Can you work these out from the model? Positions are in its coordinate system, mm. Face numbers are marked on the shaded views. A direction names the side the tool comes from. Coordinates: 2 decimals unless noted, no trailing zeros. Loops run counter-clockwise (first coordinate to the right, second up) from the corner with the lowest first, then second, coordinate; pieces in that order, holes last.
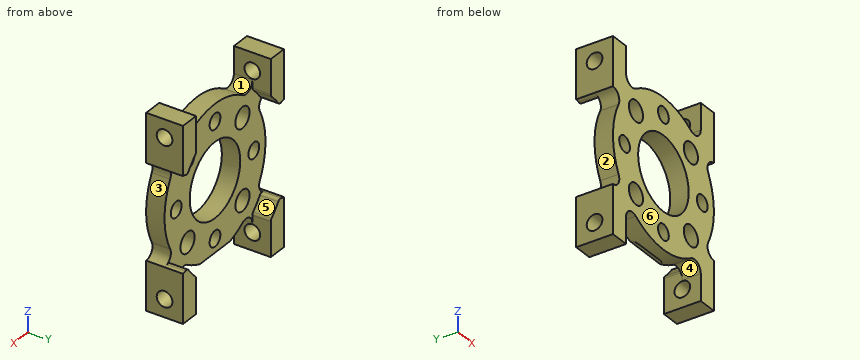
```python
from build123d import *

# Parameters (mm, degrees)
CUT_EXTRUDE1_START         = -6.35
CUT_EXTRUDE1_DEPTH         = 3.175
CUT_EXTRUDE1_START_2       = -3.175
CUT_EXTRUDE1_2_DEPTH       = 3.175
SKETCH2_W                  = 3.293618
SKETCH2_H                  = 6.35
BOSS_EXTRUDE1_DEPTH        = 4.551833731
SKETCH3_W                  = 3.293618
SKETCH3_H                  = 6.35
BOSS_EXTRUDE2_DEPTH        = 4.551833731
SKETCH4_W                  = 3.293618
SKETCH4_H                  = 6.35
BOSS_EXTRUDE3_DEPTH        = 4.551833731
SKETCH5_W                  = 3.293618
SKETCH5_H                  = 6.35
BOSS_EXTRUDE4_DEPTH        = 4.551833731
HOLE1_D                    = 12.7254
M2_5_CLEARANCE_HOLE1_D     = 2.7051
M3_CLEARANCE_HOLE1_D       = 3.556
M2_5_CLEARANCE_HOLE2_D     = 2.7051
M2_5_CLEARANCE_HOLE2_DEPTH = 3.293618
M2_5_CLEARANCE_HOLE3_D     = 2.7051
M2_5_CLEARANCE_HOLE3_DEPTH = 3.293618
M2_5_CLEARANCE_HOLE4_D     = 2.7051
M2_5_CLEARANCE_HOLE4_DEPTH = 25.4
M2_5_CLEARANCE_HOLE5_D     = 2.7051
M2_5_CLEARANCE_HOLE5_DEPTH = 3.293618
FILLET1_R                  = 0.635


with BuildPart() as part:
    # Cut-Extrude1: read off the stored shape, not the designer's step
    # Cut-Extrude1 outline → Cut-Extrude1 (new body)
    with BuildSketch(Plane(origin=(0, 6.35, 0), x_dir=(-1, 0, 0), z_dir=(0, 1, 0)).offset(CUT_EXTRUDE1_START)):
        with BuildLine():
            ThreePointArc((-12.7, 8.135112), (-11.343887812, 7.373541875), (-11.288347253, 5.819210969))
            ThreePointArc((-11.288347253, 5.819210969), (-12.7, 0), (-11.288347253, -5.819210969))
            ThreePointArc((-11.288347253, -5.819210969), (-11.343887812, -7.373541875), (-12.7, -8.135112))
            Line((-12.7, -8.135112), (-12.7, -11.958166269))
            Line((-12.7, -11.958166269), (-9.406382, -11.958166269))
            ThreePointArc((-9.406382, -11.958166269), (-8.574193969, -10.561863981), (-6.950117333, -10.629481128))
            ThreePointArc((-6.950117333, -10.629481128), (0, -12.7), (6.950117333, -10.629481128))
            ThreePointArc((6.950117333, -10.629481128), (8.574193969, -10.561863981), (9.406382, -11.958166269))
            Line((9.406382, -11.958166269), (12.7, -11.958166269))
            Line((12.7, -11.958166269), (12.7, -8.135112))
            ThreePointArc((12.7, -8.135112), (11.343887812, -7.373541875), (11.288347253, -5.819210969))
            ThreePointArc((11.288347253, -5.819210969), (12.7, 0), (11.288347253, 5.819210969))
            ThreePointArc((11.288347253, 5.819210969), (11.343887812, 7.373541875), (12.7, 8.135112))
            Line((12.7, 8.135112), (12.7, 11.958166269))
            Line((12.7, 11.958166269), (9.406382, 11.958166269))
            ThreePointArc((9.406382, 11.958166269), (8.574193969, 10.561863981), (6.950117333, 10.629481128))
            ThreePointArc((6.950117333, 10.629481128), (0, 12.7), (-6.950117333, 10.629481128))
            ThreePointArc((-6.950117333, 10.629481128), (-8.574193969, 10.561863981), (-9.406382, 11.958166269))
            Line((-9.406382, 11.958166269), (-12.7, 11.958166269))
            Line((-12.7, 11.958166269), (-12.7, 8.135112))
        make_face()
    extrude(amount=CUT_EXTRUDE1_DEPTH)

    # Cut-Extrude1 2 outline → Cut-Extrude1 2 (add)
    with BuildSketch(Plane(origin=(0, 6.35, 0), x_dir=(-1, 0, 0), z_dir=(0, 1, 0)).offset(CUT_EXTRUDE1_START_2)):
        with BuildLine():
            Line((-9.406382, 10.328643554), (-9.406382, 11.958166269))
            Line((-9.406382, 11.958166269), (-12.7, 11.958166269))
            Line((-12.7, 11.958166269), (-12.7, 8.135112))
            ThreePointArc((-12.7, 8.135112), (-12.131266538, 8.02978706), (-11.637967358, 7.727782073))
            ThreePointArc((-11.637967358, 7.727782073), (-10.602229958, 9.096901665), (-9.406382, 10.328643554))
        make_face()
        with BuildLine():
            Line((12.7, 11.958166269), (9.406382, 11.958166269))
            Line((9.406382, 11.958166269), (9.406382, 10.328643554))
            ThreePointArc((9.406382, 10.328643554), (10.602229958, 9.096901665), (11.637967358, 7.727782073))
            ThreePointArc((11.637967358, 7.727782073), (12.131266538, 8.02978706), (12.7, 8.135112))
            Line((12.7, 8.135112), (12.7, 11.958166269))
        make_face()
        with BuildLine():
            ThreePointArc((-9.406382, -10.328643554), (-10.602229958, -9.096901665), (-11.637967358, -7.727782073))
            ThreePointArc((-11.637967358, -7.727782073), (-12.131266538, -8.02978706), (-12.7, -8.135112))
            Line((-12.7, -8.135112), (-12.7, -11.958166269))
            Line((-12.7, -11.958166269), (-9.406382, -11.958166269))
            Line((-9.406382, -11.958166269), (-9.406382, -10.328643554))
        make_face()
        with BuildLine():
            ThreePointArc((12.7, -8.135112), (12.131266538, -8.02978706), (11.637967358, -7.727782073))
            ThreePointArc((11.637967358, -7.727782073), (10.602229958, -9.096901665), (9.406382, -10.328643554))
            Line((9.406382, -10.328643554), (9.406382, -11.958166269))
            Line((9.406382, -11.958166269), (12.7, -11.958166269))
            Line((12.7, -11.958166269), (12.7, -8.135112))
        make_face()
    extrude(amount=CUT_EXTRUDE1_2_DEPTH)

    # Sketch2 → Boss-Extrude1 (add)
    with BuildSketch(Plane(origin=(0, 0, -11.958166269), x_dir=(-1, 0, 0), z_dir=(0, 0, -1))):
        with Locations((11.053191, 3.175)):
            Rectangle(SKETCH2_W, SKETCH2_H)
    extrude(amount=BOSS_EXTRUDE1_DEPTH)

    # Sketch3 → Boss-Extrude2 (add)
    with BuildSketch(Plane(origin=(0, 0, -11.958166269), x_dir=(-1, 0, 0), z_dir=(0, 0, -1))):
        with Locations((-11.053191, 3.175)):
            Rectangle(SKETCH3_W, SKETCH3_H)
    extrude(amount=BOSS_EXTRUDE2_DEPTH)

    # Sketch4 → Boss-Extrude3 (add)
    with BuildSketch(Plane.XY.offset(11.958166269)):
        with Locations((11.053191, 3.175)):
            Rectangle(SKETCH4_W, SKETCH4_H)
    extrude(amount=BOSS_EXTRUDE3_DEPTH)

    # Sketch5 → Boss-Extrude4 (add)
    with BuildSketch(Plane.XY.offset(11.958166269)):
        with Locations((-11.053191, 3.175)):
            Rectangle(SKETCH5_W, SKETCH5_H)
    extrude(amount=BOSS_EXTRUDE4_DEPTH)

    # Hole1 (through all)
    with Locations(Plane(origin=(0, 3.175, 0), x_dir=(1, 0, 0), z_dir=(0, 1, 0))):
        with Locations((0, 0)):
            Hole(HOLE1_D / 2)

    # M2.5 Clearance Hole1 (through all)
    with Locations(Plane(origin=(0, 3.175, 0), x_dir=(1, 0, 0), z_dir=(0, 1, 0))):
        with Locations((0, -9.779), (-9.779, 0), (0, 9.779), (9.779, 0)):
            Hole(M2_5_CLEARANCE_HOLE1_D / 2)

    # M3 Clearance Hole1 (through all)
    with Locations(Plane(origin=(0, 3.175, 0), x_dir=(1, 0, 0), z_dir=(0, 1, 0))):
        with Locations((-6.914797213, -6.914797213), (-6.914797213, 6.914797213), (6.914797213, 6.914797213), (6.914797213, -6.914797213)):
            Hole(M3_CLEARANCE_HOLE1_D / 2)

    # M2.5 Clearance Hole2
    with Locations(Plane.ZY.offset(12.7)):
        with Locations((13.470384182, 3.175)):
            Hole(M2_5_CLEARANCE_HOLE2_D / 2, depth=M2_5_CLEARANCE_HOLE2_DEPTH)

    # M2.5 Clearance Hole3
    with Locations(Plane(origin=(-9.406382, 0, 0), x_dir=(0, 0, -1), z_dir=(1, 0, 0))):
        with Locations((13.470384182, 3.175)):
            Hole(M2_5_CLEARANCE_HOLE3_D / 2, depth=M2_5_CLEARANCE_HOLE3_DEPTH)

    # M2.5 Clearance Hole4
    with Locations(Plane(origin=(12.7, 0, 0), x_dir=(0, 0, -1), z_dir=(1, 0, 0))):
        with Locations((13.470384182, 3.175)):
            Hole(M2_5_CLEARANCE_HOLE4_D / 2, depth=M2_5_CLEARANCE_HOLE4_DEPTH)

    # M2.5 Clearance Hole5
    with Locations(Plane.ZY.offset(-9.406382)):
        with Locations((13.470384182, 3.175)):
            Hole(M2_5_CLEARANCE_HOLE5_D / 2, depth=M2_5_CLEARANCE_HOLE5_DEPTH)

    # Fillet1
    # the kernel refuses this fillet: 0.635 mm, written as the material it takes off along each edge
    with BuildSketch(Plane(origin=(-9.406382, 3.175, 10.328643554), x_dir=(0, 0, 1), z_dir=(0, 1, 0)), Plane(origin=(9.406382, 3.175, -10.328643554), x_dir=(0, 0, -1), z_dir=(0, 1, 0))) as fillet1_piece_1:
        with BuildLine():
            CenterArc((0.276858439, -0.635), FILLET1_R, 90, 46.565062077)
            ThreePointArc((-0.184250343, -0.198418174), (-0.091644431, -0.0996555), (0, 0))
            Line((0, 0), (0.276858439, 0))
        make_face()
    extrude(amount=3.867146097, mode=Mode.SUBTRACT)
    with BuildSketch(Plane(origin=(-11.637967358, 3.175, -7.727782073), x_dir=(0.5706588735868443, 0, -0.8211872198205438), z_dir=(0, 1, 0)), Plane(origin=(11.637967358, 3.175, 7.727782073), x_dir=(-0.5706588735868443, 0, 0.8211872198205438), z_dir=(0, 1, 0))) as fillet1_piece_2:
        with BuildLine():
            CenterArc((0.604132084, 0.634858067), FILLET1_R, 191.325534433, 77.463029076)
            ThreePointArc((-0.018502711, 0.51015477), (0.011380109, 0.255825664), (0, 0))
            ThreePointArc((0, 0), (0.295353463, 0.003122527), (0.590706926, 0))
        make_face()
    extrude(amount=4.651767316, mode=Mode.SUBTRACT)
    with BuildSketch(Plane(origin=(-9.406382, 3.175, -10.328643554), x_dir=(0, 0, -1), z_dir=(0, 1, 0)), Plane(origin=(9.406382, 3.175, 10.328643554), x_dir=(0, 0, 1), z_dir=(0, 1, 0))) as fillet1_piece_3:
        with BuildLine():
            CenterArc((0.276858439, 0.635), FILLET1_R, 223.434937923, 46.565062077)
            ThreePointArc((-0.184250343, 0.198418174), (-0.091644431, 0.0996555), (0, 0))
            Line((0, 0), (0.276858439, 0))
        make_face()
    extrude(amount=3.867146097, mode=Mode.SUBTRACT)
    with BuildSketch(Plane(origin=(-11.637967358, 3.175, 7.727782073), x_dir=(0.5706588735868457, 0, 0.8211872198205425), z_dir=(0, 1, 0)), Plane(origin=(11.637967358, 3.175, -7.727782073), x_dir=(-0.5706588735868457, 0, -0.8211872198205425), z_dir=(0, 1, 0))) as fillet1_piece_4:
        with BuildLine():
            CenterArc((0.604132084, -0.634858067), FILLET1_R, 91.211436491, 77.463029076)
            ThreePointArc((-0.018502711, -0.51015477), (0.011380109, -0.255825664), (0, 0))
            ThreePointArc((0, 0), (0.295353463, -0.003122527), (0.590706926, 0))
        make_face()
    extrude(amount=4.651767316, mode=Mode.SUBTRACT)


solid = part.part
```
(1) I'm going to push a flat-ended pin straight in: pin 1 (3 mm diameter, centred on y = 3.5, z = -4, fed in from +X). Where does the tip first touch, or does it pass through?
Check values:
pin 1: stops at x = 12.44
(2) I want a section at B-B on y = 5.75. Write out the boundary of the cut face in (x, z) (1 decimal).
Check values:
outline: (-12.7, -16.5) - (-9.4, -16.5) - (-9.4, -10.6) arc R0.6 ccw to (-9.6, -10.1) arc R14 cw to (-11.3, -8.2) arc R0.6 ccw to (-12.1, -8) arc R1.6 cw to (-12.7, -8.1) - close; (-12.7, 8.1) arc R1.6 cw to (-12.1, 8) arc R0.6 ccw to (-11.3, 8.2) arc R14 cw to (-9.6, 10.1) arc R0.6 ccw to (-9.4, 10.6) - (-9.4, 16.5) - (-12.7, 16.5) - close; (9.4, -16.5) - (12.7, -16.5) - (12.7, -8.1) arc R1.6 cw to (12.1, -8) arc R0.6 ccw to (11.3, -8.2) arc R14 cw to (9.6, -10.1) arc R0.6 ccw to (9.4, -10.6) - close; (9.4, 10.6) arc R0.6 ccw to (9.6, 10.1) arc R14 cw to (11.3, 8.2) arc R0.6 ccw to (12.1, 8) arc R1.6 cw to (12.7, 8.1) - (12.7, 16.5) - (9.4, 16.5) - close
(3) Which directions (+Z, -Z, +X, -X, +Y, -Y) give clear straight access to the entire face, cutting with the end or side of a thin tool? Please do the marked faces 5 and 6.
Check values:
face 5: +Y
face 6: +Z, -Z, +X, -X, -Y
(4) If I drill on probe 1 along X at (y, z) = (4.75, 14.5); probe 2 along Y at (x, z) = (-11, 13.5); probe 3 along Z at (x, y) = (-8.25, 2.5), over which ranges is the centre line in solid material (lowest first)?
Check values:
probe 1: x = -12.7 to -9.41, 9.41 to 12.7
probe 2: y = 0 to 1.82, 4.53 to 6.35
probe 3: z = -10.43 to -8.09, -5.74 to 5.74, 8.09 to 10.43
(5) If we mould it in two halves opening along Z, with no side actions, what happens to the marked faces 1, 2, 3 and 4? For each: released by +Z, released by -Z, zero draft, split by the parting line, or undercut.
Check values:
face 1: released by +Z
face 2: undercut
face 3: undercut
face 4: released by -Z
(6) I want a section at A-A on z = 0. Write out the boundary of the cut face in (x, y) (3 decimals).
Check values:
outline: (-12.7, 0) - (-11.132, 0) - (-11.132, 3.175) - (-12.7, 3.175) - close; (-8.426, 0) - (-6.363, 0) - (-6.363, 3.175) - (-8.426, 3.175) - close; (6.363, 0) - (8.426, 0) - (8.426, 3.175) - (6.363, 3.175) - close; (11.132, 0) - (12.7, 0) - (12.7, 3.175) - (11.132, 3.175) - close
(7) I want a section at C-C on x = 0. Write out the boundary of the cut face in (y, z) (3 decimals).
Check values:
outline: (0, -12.7) - (2.063, -12.7) arc R1.353 cw to (3.175, -12.118) - (3.175, -11.132) - (0, -11.132) - close; (0, -8.426) - (3.175, -8.426) - (3.175, -6.363) - (0, -6.363) - close; (0, 6.363) - (3.175, 6.363) - (3.175, 8.426) - (0, 8.426) - close; (0, 11.132) - (3.175, 11.132) - (3.175, 12.7) - (0, 12.7) - close
(8) I want a section at D-D on x = 4.25. Write out the boundary of the cut face in (y, z) (3 decimals).
Check values:
outline: (0, -11.968) - (3.175, -11.968) - (3.175, -4.735) - (0, -4.735) - close; (0, 4.735) - (3.175, 4.735) - (3.175, 11.968) - (0, 11.968) - close
